```python
from build123d import *

# Parameters (mm, degrees)
ESQUISSE1_R             = 3.5
BASE_EXTRUSION_DEPTH    = 22
ESQUISSE2_W             = 37.834703774
ESQUISSE2_H             = 34.90934008
ENL_V_MAT_EXTRU_1_DEPTH = 6
ESQUISSE3_R             = 3.5
ENL_V_MAT_EXTRU_2_DEPTH = 91.245498503


with BuildPart() as part:
    # Esquisse1 → Base-Extrusion (new body)
    with BuildSketch(Plane(origin=(0, 0, 0), x_dir=(-1, 0, 0), z_dir=(0, 0, -1))):
        Polygon((12.5, -12.5), (-5.17766953, -12.5), (-23, 5.32233047), (-23, 56), (-29, 62), (-29, 74), (-23, 80), (-11, 80), (-5, 74), (-5, 28.864908166), (12.5, 3.951485697), align=None)
        with Locations(Location((0, 0, 0), (0, 0, 90))):
            Circle(ESQUISSE1_R, mode=Mode.SUBTRACT)
        with Locations(Location((-17, 71, 0), (0, 0, 90))):
            Circle(ESQUISSE1_R, mode=Mode.SUBTRACT)
    extrude(amount=BASE_EXTRUSION_DEPTH)

    # Esquisse2 → Enlèv. mat.-Extru.1 (cut, symmetric)
    with BuildSketch(Plane.XY.offset(-11)):
        with Locations((15.075848619, 69.45467004)):
            Rectangle(ESQUISSE2_W, ESQUISSE2_H)
    extrude(amount=ENL_V_MAT_EXTRU_1_DEPTH, both=True, mode=Mode.SUBTRACT)

    # Esquisse3 → Enlèv. mat.-Extru.2 (cut, through all)
    with BuildSketch(Plane(origin=(23, 0, 0), x_dir=(0, 0, -1), z_dir=(1, 0, 0))):
        with Locations(Location((11, 35, 0), (0, 0, 90))):
            Circle(ESQUISSE3_R)
    extrude(amount=-ENL_V_MAT_EXTRU_2_DEPTH, mode=Mode.SUBTRACT)


solid = part.part
```
Work out the finished part from the listing and answer in its coordinate system (mm). A direction names the side the tool comes from. Give positions to 0.01 mm unless a question says otherwise; leave off trailing zeros. Loops run counter-clockwise (first coordinate to the right, second up) from the corner with the lowest first, then second, coordinate; pieces in that order, holes last. Notation, with made-up numbers: M 0,-3 L 12,-3 A25 ccw 12,21 Z; hole C 20.5,33.5 d11. An arc over 180 degrees is marked long. One line per item, written item: value. Start each with the question number.
1. Find the intervals of material crossed by probe 1 along Z at (x, y) = (6.5, 69); probe 2 along X at (y, z) = (71, -2.9); probe 3 along Z at (x, y) = (17, 35), in increasing order.
2. Find section B-B (z = -15.5). Give the vertices of the cut face in (x, y), and give its area (3 significant figures).
3. Which of the six approach directions +Z, -Z, +X, -X, +Y, -Y give full straight-line access (tool end or side, diameter ignored) to faces 1 (the face through (5, 47, -11)), 2 (the face through (14, 52, -11)), 3 (the face through (19.365, 68.42, -2.465))?
4. Find section C-C (x = 17). Give the vertices of the cut face in (y, z).
5. Find section A-A (y = 35). Give the vertices of the cut face in (x, z), and give its area (3 significant figures).
6. Determine the mould class of faces 4 (the face through (13, 34, -22)), 5 (the face through (14.126, 31.503, -10.846)), 6 (the face through (26, 59, -19)) for opening direction Z: released by +Z, released by -Z, zero draft, split by the parting line, or undercut.
7. Each of these flat-tipped pins is pushed along its axis until it touches: P1, Ø9, axis at y = 35, z = -11, coming from the +X side; P2, Ø3, axis at x = 7.5, z = -13.5, coming from the +Y side; P3, Ø11, axis at y = 55.5, z = -8, coming from the -X side. Where does it stop, or does it pass through?
8. Find section D-D (z = -20.25). Give the vertices of the cut face in (x, y).
Reported:
1. probe 1: z = -22 to -17, -5 to 0
1. probe 2: x = 5 to 13.5, 20.5 to 29
1. probe 3: z = -22 to -14.5, -7.5 to 0
2. outline: M -12.5,-12.5 L 5.18,-12.5 L 23,5.32 L 23,52 L 5,52 L 5,28.86 L -12.5,3.95 Z; hole C 0,0 d7
2. area: 1,470 mm²
3. face 1: +Z, -Z, -X, +Y
3. face 2: +X, -X, +Y
3. face 3: +Z, -Z
4. outline: M -0.68,-22 L 67.5,-22 L 67.5,-17 L 52,-17 L 52,-5 L 67.5,-5 L 67.5,0 L -0.68,0 Z; M 74.5,-22 L 80,-22 L 80,-17 L 74.5,-17 Z; M 74.5,-5 L 80,-5 L 80,0 L 74.5,0 Z; hole C 35,-11 d7
5. outline: M 5,-22 L 23,-22 L 23,-14.5 L 5,-14.5 Z; M 5,-7.5 L 23,-7.5 L 23,0 L 5,0 Z
5. area: 270 mm²
6. face 4: released by -Z
6. face 5: undercut
6. face 6: zero draft
7. P1: stops at x = 23
7. P2: stops at y = 52
7. P3: stops at x = 5
8. outline: M -12.5,-12.5 L 5.18,-12.5 L 23,5.32 L 23,56 L 29,62 L 29,74 L 23,80 L 11,80 L 5,74 L 5,28.86 L -12.5,3.95 Z; hole C 0,0 d7; hole C 17,71 d7
